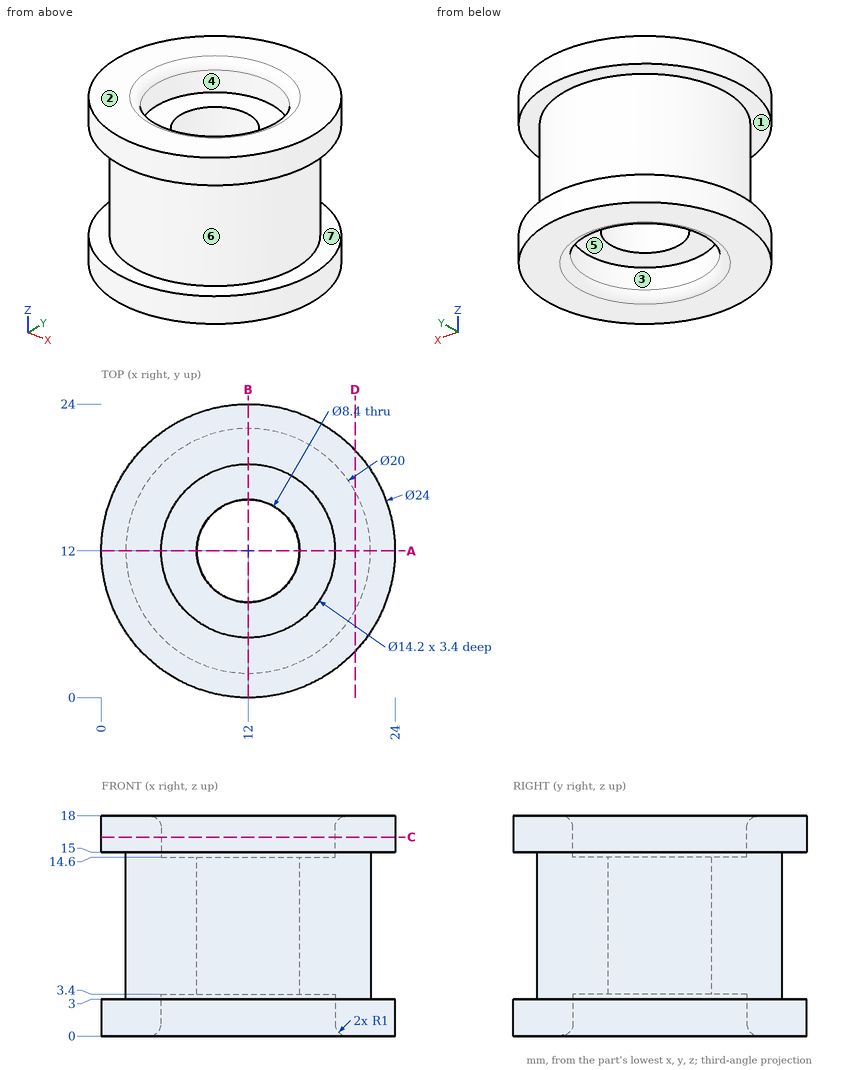
Here's the drawing with two shaded views (mm, measured from the low corner). I have some questions. A direction names the side the tool comes from. Coordinates: 2 decimals unless noted, no trailing zeros. Order: outer loops, then holes, each group sorted by start corner. A loop starts at its lowest first (then second) coordinate and runs counter-clockwise, first axis right, second up. Notation, with made-up numbers: (3.5, 79) -> (32.5, 79) arc R23 ccw to (32.5, 118) -> close; hole circle Ø7 at (-5.5, 64.5). An arc over 180 degrees is marked (long way). Write each question's results on one line, items separated by ' | '.
Item 1: I want a section at D-D, the plane x = 20.75. Write out the boundary of the cut face in (y, z).
Results are:
outline: (3.79, 0) -> (20.21, 0) -> (20.21, 3) -> (16.84, 3) -> (16.84, 15) -> (20.21, 15) -> (20.21, 18) -> (3.79, 18) -> (3.79, 15) -> (7.16, 15) -> (7.16, 3) -> (3.79, 3) -> close
Item 2: If we mould it in two halves opening along X, with no side actions, what happens to the marked faces 5, 6 and 7? For each: +X half, -X half, draft (parallel to the pull), parting line (faces both ways), or undercut.
Results are:
face 5: undercut | face 6: parting line | face 7: draft
Item 3: I'm going to push flat-ended pins straight in: pin 1 Ø1.5 at (x, z) = (5.5, 9.5) entering from -Y; pin 2 Ø3 at (x, z) = (14.5, 10) entering from +Y; pin 3 Ø13 at (x, y) = (12, 12) entering from -Z. Where does each tip first touch, or does it pass through?
Results are:
pin 1: y = 3.82 | pin 2: y = 21.95 | pin 3: z = 3.4
Item 4: Which directions (+Z, -Z, +X, -X, +Y, -Y) give clear straight access to the entire face, cutting with the end or side of a thin tool? Please do the marked faces 1, 2, 3 and 4.
Results are:
face 1: none | face 2: +Z, +X, -X, +Y, -Y | face 3: -Z | face 4: +Z
Item 5: If I drill on line 1 along Y through (x, z) = (12, 1.75); line 2 along Z through (x, y) = (16.5, 2.75); line 3 along X through (y, z) = (11.75, 10.25), over which ranges is the centre line in solid material (lowest first)?
Results are:
line 1: 0 to 4.9, 19.1 to 24 | line 2: 0 to 3, 15 to 18 | line 3: 2 to 7.81, 16.19 to 22
Item 6: I want a section at A-A, the plane y = 12. Write out the boundary of the cut face in (x, z).
Results are:
outline: (0, 0) -> (3.9, 0) arc R1 ccw to (4.9, 1) -> (4.9, 3.4) -> (7.8, 3.4) -> (7.8, 14.6) -> (4.9, 14.6) -> (4.9, 17) arc R1 ccw to (3.9, 18) -> (0, 18) -> (0, 15) -> (2, 15) -> (2, 3) -> (0, 3) -> close; (16.2, 3.4) -> (19.1, 3.4) -> (19.1, 1) arc R1 ccw to (20.1, 0) -> (24, 0) -> (24, 3) -> (22, 3) -> (22, 15) -> (24, 15) -> (24, 18) -> (20.1, 18) arc R1 ccw to (19.1, 17) -> (19.1, 14.6) -> (16.2, 14.6) -> close
Item 7: I want a section at C-C, the plane z = 16.25. Write out the boundary of the cut face in (x, y), then the cut area to 3 significant figures.
Results are:
outline: circle Ø24 at (12, 12); hole circle Ø14.2 at (12, 12) | area: 294 mm²
